Source: CAD feature listing. Evaluate the final solid. Frame: model axes, mm. A direction names the side the tool comes from. Coordinates: 2 decimals unless noted, no trailing zeros. Write each loop counter-clockwise with the first axis right and the second up, starting at its lowest first coordinate (ties: lowest second). Pieces come first, ordered by that corner, then holes. Notation, with made-up numbers: (-16, -3) - (-3, -3) arc R23 cw to (-3, 31) - close; hole circle Ø10 at (7.25, -12). An arc over 180 degrees is marked (long way). One line per question, with ' | ' between items. Start each with the question number.
Q1. Draft query along Y for faces 1 (the face through (52.617, -15.028, 12.495)), 2 (the face through (2, 40, 76.2)), 3 (the face through (53.97, 17.98, 11.06)). Return one class per face: +Y half, -Y half, draft (parallel to the pull), parting line (faces both ways), or undercut.
Q2. Cut plane A-A, the plane z = 67. Return loops of the section in (x, y).
Q3. Cut plane C-C, the plane z = 22. Return loops of the section in (x, y).
Q4. Contact query for flat-ended pins moving along their axis: P1, Ø3, axis at x = 38, y = -11.5, coming from the -Z side; P2, Ø23.5, axis at x = 8.5, y = -1.5, coming from the +Z side; P3, Ø3, axis at x = -41.5, y = -26, coming from the -Z side. Output: stop coordinate, or through.
Q5. Line query: line 1 (Y direction, x = 30.5, z = 43.5); line 2 (Y direction, x = -19, z = 17); line 3 (X direction, y = 34.5, z = 55). Output: solid intervals per line, ascending.
Q6. Cut plane B-B, the plane x = -11. Return loops of the section in (y, z), plus the area to 3 significant figures.
Q7. Access query for faces 4 (the face through (3.295, 32.206, 9.414)), 5 (the face through (-53.82, -19.055, 50.444)). Directions: +Z, -Z, +X, -X, +Y, -Y. A direction counts if a zero-diameter tool reaches every point of the face in a straight line with its end or side. Return the directions, or none.
```python
from build123d import *

# Parameters (mm, degrees)
F1_DEPTH = 76.2
F2_R     = 25.4
F3_T     = -2.54


with BuildPart() as f1:
    # F0 (on Top) → F1 (new body)
    with BuildSketch(Plane.XY):
        Polygon((-31.621649, 41.264485), (-70.740356, 0), (-36.419954, -38.650967), (39.222521, -38.650967), (75.863615, 0), (39.222521, 41.264485), align=None)
    extrude(amount=F1_DEPTH)

    # F2
    f2_edges = [f1.edges().sort_by_distance(p)[0] for p in [
        (3.800436, 41.264485, 0),
        (-51.181002, 20.632243, 0),
        (-53.580155, -19.325484, 0),
        (1.401283, -38.650967, 0),
        (57.543068, -19.325484, 0),
        (57.543068, 20.632243, 0),
    ]]
    fillet(f2_edges, radius=F2_R)

    # F3
    f3_openings = [f1.faces().sort_by_distance(p)[0] for p in [
        (2.587769, 0.870708, 76.2),
    ]]
    offset(amount=F3_T, openings=f3_openings)


solid = f1.part
```
Reply:
1) face 1: undercut | face 2: draft | face 3: +Y half
2) outline: (-70.74, 0) - (-36.42, -38.65) - (39.22, -38.65) - (75.86, 0) - (39.22, 41.26) - (-31.62, 41.26) - close; hole (-67.29, -0.06) - (-35.28, -36.11) - (38.13, -36.11) - (72.42, 0.06) - (38.08, 38.72) - (-30.53, 38.72) - close
3) outline: (-70.43, -0.01) - (-36.32, -38.42) - (39.12, -38.42) - (75.55, 0.01) - (39.12, 41.04) - (-31.52, 41.04) - close; hole (-66.95, -0.06) - (-35.16, -35.86) - (38.02, -35.86) - (72.07, 0.06) - (37.97, 38.47) - (-30.42, 38.47) - close
4) P1: stops at z = 0.37 | P2: stops at z = 2.54 | P3: stops at z = 8.89
5) line 1: y = -38.65 to -36.11, 38.72 to 41.26 | line 2: y = -37.22 to -34.51, 37.13 to 39.84 | line 3: x = -38.03 to -34.53, 41.83 to 45.23
6) outline: (-38.65, 25.4) arc R25.4 ccw to (-13.25, 0) - (15.86, 0) arc R25.4 ccw to (41.26, 25.4) - (41.26, 76.2) - (38.72, 76.2) - (38.72, 25.4) arc R22.86 cw to (15.86, 2.54) - (-13.25, 2.54) arc R22.86 cw to (-36.11, 25.4) - (-36.11, 76.2) - (-38.65, 76.2) - close | area: 525 mm^2
7) face 4: +Z | face 5: +Z, -Z, -X, -Y
